from build123d import *

# Parameters (mm, degrees)
SKETCH1_W           = 292.1
SKETCH1_H           = 139.7
BOSS_EXTRUDE1_DEPTH = 9.525
SKETCH2_W           = 33.02
SKETCH2_H           = 25.4
CUT_EXTRUDE1_DEPTH  = 9.525
SKETCH3_R           = 3.175
CUT_EXTRUDE2_DEPTH  = 9.525
SKETCH4_W           = 25.4
SKETCH4_H           = 12.7
BOSS_EXTRUDE2_DEPTH = 20.32
SKETCH5_W           = 25.4
SKETCH5_H           = 10.16
CUT_EXTRUDE3_DEPTH  = 17.78
FILLET2_R           = 7.62
SKETCH6_R           = 6.35
CUT_EXTRUDE4_DEPTH  = 2.54


with BuildPart() as part:
    # Sketch1 → Boss-Extrude1 (new body)
    with BuildSketch(Plane(origin=(0, 0, 0), x_dir=(1, 0, 0), z_dir=(0, 1, 0))):
        Rectangle(SKETCH1_W, SKETCH1_H)
    extrude(amount=BOSS_EXTRUDE1_DEPTH)

    # Sketch2 → Cut-Extrude1 (cut)
    with BuildSketch(Plane(origin=(0, 9.525, 0), x_dir=(1, 0, 0), z_dir=(0, 1, 0))):
        with Locations((-120.015, 46.99)):
            Rectangle(SKETCH2_W, SKETCH2_H)
        with Locations((-120.015, -46.99)):
            Rectangle(SKETCH2_W, SKETCH2_H)
        with Locations((120.015, 46.99)):
            Rectangle(SKETCH2_W, SKETCH2_H)
        with Locations((120.015, -46.99)):
            Rectangle(SKETCH2_W, SKETCH2_H)
    extrude(amount=-CUT_EXTRUDE1_DEPTH, mode=Mode.SUBTRACT)

    # Sketch3 → Cut-Extrude2 (cut)
    with BuildSketch(Plane(origin=(146.05, 0, 0), x_dir=(0, 0, -1), z_dir=(1, 0, 0))):
        with Locations((-46.99, 4.7625)):
            Circle(SKETCH3_R)
        with Locations((46.99, 4.7625)):
            Circle(SKETCH3_R)
    cut_extrude2 = extrude(amount=-CUT_EXTRUDE2_DEPTH, mode=Mode.SUBTRACT)

    # Mirror1: Cut-Extrude2 across plane
    add(cut_extrude2.mirror(Plane(origin=(0, 0, 0), x_dir=(0, 0, 1), z_dir=(1, 0, 0))), mode=Mode.SUBTRACT)

    # Sketch4 → Boss-Extrude2 (add)
    with BuildSketch(Plane(origin=(0, 9.525, 0), x_dir=(1, 0, 0), z_dir=(0, 1, 0))):
        with Locations((88.9, 62.590737259)):
            Rectangle(SKETCH4_W, SKETCH4_H)
    extrude(amount=BOSS_EXTRUDE2_DEPTH)

    # Sketch5 → Cut-Extrude3 (cut)
    with BuildSketch(Plane(origin=(0, 29.845, 0), x_dir=(1, 0, 0), z_dir=(0, 1, 0))):
        with Locations((88.9, 61.320737259)):
            Rectangle(SKETCH5_W, SKETCH5_H)
    extrude(amount=-CUT_EXTRUDE3_DEPTH, mode=Mode.SUBTRACT)

    # Fillet2
    fillet2_edges = [part.edges().sort_by_distance(p)[0] for p in [
        (101.6, 29.845, -67.670737259),
        (76.2, 29.845, -67.670737259),
    ]]
    fillet(fillet2_edges, radius=FILLET2_R)

    # Sketch6 → Cut-Extrude4 (cut)
    with BuildSketch(Plane(origin=(0, 0, -68.940737259), x_dir=(-1, 0, 0), z_dir=(0, 0, -1))):
        with Locations((-88.9, 19.685)):
            Circle(SKETCH6_R)
    extrude(amount=-CUT_EXTRUDE4_DEPTH, mode=Mode.SUBTRACT)


solid = part.part
Could you check a few things on this model? Use its own coordinates, in mm. A direction names the side the tool comes from. Coordinates: 2 decimals unless noted, no trailing zeros. Write each loop counter-clockwise with the first axis right and the second up, starting at its lowest first coordinate (ties: lowest second). Pieces come first, ordered by that corner, then holes. Notation, with made-up numbers: (68.25, 78) - (118.25, 78) arc R22 ccw to (118.25, 117) - close; hole circle Ø4 at (74, 88). An arc over 180 degrees is marked (long way). Put each result on its own line as item: value. Start each with the question number.
Q1. I'm going to push flat-ended pins straight in: P1, Ø3, axis at x = 83, y = 26, coming from the -Z side; P2, Ø1.5, axis at x = -22.5, z = 45, coming from the +Y side (3 decimals); P3, Ø9, axis at x = 84, y = 19, coming from the +Z side. Where does each tip first touch, or does it pass through?
Q2. Which directions (+Z, -Z, +X, -X, +Y, -Y) give clear straight access to the entire face, cutting with the end or side of a thin tool? Please do faces 1 (the cylindrical face through (-141.354, 3.546, 44.057)), 2 (the flat face through (101.6, 11.6, -65.3)), 3 (the flat face through (83, 23, -66.401)), 4 (the flat face through (-120, 5, 59.69)).
Q3. Please list where these lines run through material, in increasing order: L1, parallel to X at y = 2, z = -59 (3 decimals); L2, parallel to Y at x = 88, z = -67 (3 decimals); L3, parallel to Y at x = -139.5, z = 46.99 (1 decimal).
Q4. I want a section at D-D on x = -100. Write out the boundary of the cut face in (y, z) (3 decimals).
Q5. Thinking about a two-plate mould opening in X: for faces 5 (the flat face through (76.2, 11.6, -65.3)), 6 (the cylindrical face through (141.354, 3.546, 44.057)), 7 (the flat face through (120, 5, 34.29)), which applies, pulls with the +X half, pulls with the -X half, needs draft (parallel to the pull), parting line crosses it, or undercut?
Q6. I want a section at A-A on x = 88.9. Write out the boundary of the cut face in (y, z) (3 decimals), plus the area to 3 significant figures.
Q7. I want a section at B-B on z = -46.99. Count the separate pieces of the cut face and the enclosed holes in it, plus the area to 3 significant figures.
Q8. I want a section at C-C on z = 16.5. Write out the boundary of the cut face in (x, y) (3 decimals).
Checks:
1. P1: z = -68.94
1. P2: y = 9.525
1. P3: z = -66.4
2. face 1: -X
2. face 2: +Z, -Z, +X, +Y
2. face 3: +Z, +X, -X, +Y
2. face 4: +Y, -Y
3. L1: -146.05 to -136.525, -103.505 to 103.505, 136.525 to 146.05
3. L2: 0 to 13.399, 25.971 to 29.845
3. L3: 0 to 1.6, 7.9 to 9.5
4. outline: (0, -69.85) - (9.525, -69.85) - (9.525, 69.85) - (0, 69.85) - close
5. face 5: pulls with the -X half
5. face 6: needs draft
5. face 7: undercut
6. outline: (0, -69.85) - (9.525, -69.85) - (9.525, -68.941) - (13.335, -68.941) - (13.335, -66.401) - (12.065, -66.401) - (12.065, -56.241) - (9.525, -56.241) - (9.525, 69.85) - (0, 69.85) - close; (26.035, -68.941) - (29.845, -68.941) - (29.845, -66.401) - (26.035, -66.401) - close
6. area: 1,380 mm²
7. separate pieces: 5
7. enclosed holes: 0
7. area: 2,030 mm²
8. outline: (-146.05, 0) - (146.05, 0) - (146.05, 9.525) - (-146.05, 9.525) - close
